Autodesk Inventor part; units mm, degrees
ref_plane "YZ Plane" through (0, 0, 0) normal (1, 0, 0) x (0, 1, 0)
ref_plane "XZ Plane" through (0, 0, 0) normal (0, 1, 0) x (-1, 0, 0)
ref_plane "XY Plane" through (0, 0, 0) normal (0, 0, 1) x (1, 0, 0)
sketch "Sketch1" plane through (0, 0, 0) normal (0, 0, 1) x (1, 0, 0)
  circle A0 centre (0, 0) radius 7.5
  line L0 (-16, 7.5) -> (16, 7.5)
  line L1 (16, 7.5) -> (16, -9.5)
  line L2 (16, -9.5) -> (-16, -9.5)
  line L3 (-16, -9.5) -> (-16, 7.5)
  line L4 (-7.5, 0) -> (-7.5, 7.5)
  line L5 (7.5, 0) -> (7.5, 7.5)
  point P0 (0, -9.5)
  dimension "d0" = 15
  dimension "d5" = 32
  dimension "d6" = 2
extrude "Extrusion1" add sketch "Sketch1" along normal blind 24.2 contours A0 L5 L0 L1 L2 L3 L4
sketch "Sketch2" plane through (0, 0, 24.2) normal (0, 0, 1) x (1, 0, 0)
  line L0 (-16, -9.5) -> (16, -9.5)
  line L1 (16, -9.5) -> (16, 7.5)
  line L2 (16, 7.5) -> (7.5, 7.5)
  line L3 (7.5, 7.5) -> (7.5, 0)
  arc A0 (-7.5, 0) -> (7.5, 0) centre (0, 0) ccw
  line L4 (-7.5, 0) -> (-7.5, 7.5)
  line L5 (-7.5, 7.5) -> (-16, 7.5)
  line L6 (-16, 7.5) -> (-16, -9.5)
  circle A1 centre (0, 0) radius 4.25
  line L7 (-7.5, 7.5) -> (-16, 7.5)
  line L8 (-7.5, 7.5) -> (7.5, 7.5)
  dimension "d10" = 8.5
extrude "Extrusion3" add sketch "Sketch2" along normal blind 3
sketch "Sketch4" plane through (0, 0, 0) normal (0, 0, -1) x (-1, 0, 0)
  line L0 (-16, 7.5) -> (-7.5, 7.5)
  line L1 (-16, -9.5) -> (-16, 7.5)
  line L2 (16, -9.5) -> (-16, -9.5)
  line L3 (16, 7.5) -> (16, -9.5)
  line L4 (7.5, 7.5) -> (16, 7.5)
  line L5 (-7.5, 7.5) -> (7.5, 7.5)
  circle A0 centre (0, 0) radius 4.25
extrude "Extrusion4" add sketch "Sketch4" along normal blind 3
sketch "Sketch5" plane through (0, 0, -3) normal (0, 0, -1) x (-1, 0, 0)
  line L0 (16, 7.5) -> (-16, 7.5)
  line L1 (16, -9.5) -> (16, 7.5)
  line L2 (-16, -9.5) -> (16, -9.5)
  line L3 (-16, 7.5) -> (-16, -9.5)
  circle A0 centre (0, 0) radius 7.5
  arc A1 (-7.5, 0) -> (7.5, 0) centre (0, 0) ccw
  line L4 (7.5, 0) -> (7.5, 7.5)
  line L5 (-16, 7.5) -> (16, 7.5)
  line L6 (-7.5, 7.5) -> (-7.5, 0)
  line L7 (-7.5, 0) -> (-7.5, 7.5)
extrude "Extrusion5" add sketch "Sketch5" along normal blind 130 contours L1 L2 L3 L0 L6 A0 L4
sketch "Sketch6" plane through (0, 0, -133) normal (0, 0, -1) x (-1, 0, 0)
  line L0 (0, 0) -> (0, -9.5) construction
  line L1 (16, -9.5) -> (-16, -9.5) construction
  line L2 (-16, 7.5) -> (-16, -9.5) construction
  point P0 (-12.5, -6)
  point P1 (12.5, -6)
  dimension "d17" = 3.5
  dimension "d18" = 3.5
hole "Hole1" at (12.5, -6, -133) at (-12.5, -6, -133) direction (0, 0, 1) diameter 2.3813 depth 10 tip angle 118
sketch "Sketch7" plane through (-16, 7.5, 27.2) normal (0, 1, 0) x (1, 0, 0)
  line L0 (16, 0) -> (16, 160.2) construction
  line L1 (32, 160.2) -> (0, 160.2)
  line L2 (0, 160.2) -> (0, 0)
  line L3 (32, 0) -> (0, 0)
  point P0 (16, 27.2)
  point P1 (3.5, 3.5)
  point P2 (3.5, 33.5)
  point P3 (3.5, 63.5)
  point P4 (3.5, 93.5)
  point P5 (3.5, 123.5)
  point P6 (3.5, 145.2)
  point P7 (28.5, 3.5)
  point P8 (28.5, 33.5)
  point P9 (28.5, 63.5)
  point P10 (28.5, 93.5)
  point P11 (28.5, 123.5)
  point P12 (28.5, 145.2)
  dimension "d27" = 3.5
  dimension "d44" = 30
  dimension "d49" = 3.5
  dimension "d50" = 15
hole "Hole3" at (-12.5, 7.5, 23.7) at (-12.5, 7.5, -6.3) at (-12.5, 7.5, -36.3) at (-12.5, 7.5, -66.3) at (-12.5, 7.5, -96.3) at (-12.5, 7.5, -118) at (12.5, 7.5, 23.7) at (12.5, 7.5, -6.3) at (12.5, 7.5, -36.3) at (12.5, 7.5, -66.3) at (12.5, 7.5, -96.3) at (12.5, 7.5, -118) direction (0, -1, 0) diameter 3.175 end through all
sketch "Sketch8" plane through (-16, -9.5, 27.2) normal (0, -1, 0) x (1, 0, 0)
  circle A0 centre (28.5, -3.5) radius 1.5875
  line L0 (30.2321, -6.5) -> (26.7679, -6.5)
  line L1 (26.7679, -6.5) -> (25.0359, -3.5)
  line L2 (25.0359, -3.5) -> (26.7679, -0.5)
  line L3 (26.7679, -0.5) -> (30.2321, -0.5)
  line L4 (30.2321, -0.5) -> (31.9641, -3.5)
  line L5 (31.9641, -3.5) -> (30.2321, -6.5)
  line L6 (5.2321, -6.5) -> (1.7679, -6.5)
  line L7 (1.7679, -0.5) -> (5.2321, -0.5)
  line L8 (5.2321, -0.5) -> (6.9641, -3.5)
  line L9 (6.9641, -3.5) -> (5.2321, -6.5)
  line L10 (1.7679, -6.5) -> (0.0359, -3.5)
  line L11 (0.0359, -3.5) -> (1.7679, -0.5)
  line L12 (0, 0) -> (0, -160.2)
  line L13 (1.7679, -36.5) -> (0.0359, -33.5)
  line L14 (0.0359, -33.5) -> (1.7679, -30.5)
  line L15 (1.7679, -30.5) -> (5.2321, -30.5)
  line L16 (5.2321, -30.5) -> (6.9641, -33.5)
  line L17 (6.9641, -33.5) -> (5.2321, -36.5)
  line L18 (25.0359, -33.5) -> (26.7679, -30.5)
  line L19 (26.7679, -36.5) -> (25.0359, -33.5)
  line L20 (30.2321, -36.5) -> (26.7679, -36.5)
  line L21 (31.9641, -33.5) -> (30.2321, -36.5)
  line L22 (30.2321, -30.5) -> (31.9641, -33.5)
  line L23 (26.7679, -30.5) -> (30.2321, -30.5)
  line L24 (1.7679, -66.5) -> (0.0359, -63.5)
  line L25 (0.0359, -63.5) -> (1.7679, -60.5)
  line L26 (1.7679, -60.5) -> (5.2321, -60.5)
  line L27 (5.2321, -60.5) -> (6.9641, -63.5)
  line L28 (6.9641, -63.5) -> (5.2321, -66.5)
  line L29 (25.0359, -63.5) -> (26.7679, -60.5)
  line L30 (26.7679, -66.5) -> (25.0359, -63.5)
  line L31 (30.2321, -66.5) -> (26.7679, -66.5)
  line L32 (31.9641, -63.5) -> (30.2321, -66.5)
  line L33 (30.2321, -60.5) -> (31.9641, -63.5)
  line L34 (26.7679, -60.5) -> (30.2321, -60.5)
  line L35 (1.7679, -96.5) -> (0.0359, -93.5)
  line L36 (0.0359, -93.5) -> (1.7679, -90.5)
  line L37 (1.7679, -90.5) -> (5.2321, -90.5)
  line L38 (5.2321, -90.5) -> (6.9641, -93.5)
  line L39 (6.9641, -93.5) -> (5.2321, -96.5)
  line L40 (25.0359, -93.5) -> (26.7679, -90.5)
  line L41 (26.7679, -96.5) -> (25.0359, -93.5)
  line L42 (30.2321, -96.5) -> (26.7679, -96.5)
  line L43 (31.9641, -93.5) -> (30.2321, -96.5)
  line L44 (30.2321, -90.5) -> (31.9641, -93.5)
  line L45 (26.7679, -90.5) -> (30.2321, -90.5)
  line L46 (1.7679, -126.5) -> (0.0359, -123.5)
  line L47 (0.0359, -123.5) -> (1.7679, -120.5)
  line L48 (1.7679, -120.5) -> (5.2321, -120.5)
  line L49 (5.2321, -120.5) -> (6.9641, -123.5)
  line L50 (6.9641, -123.5) -> (5.2321, -126.5)
  line L51 (25.0359, -123.5) -> (26.7679, -120.5)
  line L52 (26.7679, -126.5) -> (25.0359, -123.5)
  line L53 (30.2321, -126.5) -> (26.7679, -126.5)
  line L54 (31.9641, -123.5) -> (30.2321, -126.5)
  line L55 (30.2321, -120.5) -> (31.9641, -123.5)
  line L56 (26.7679, -120.5) -> (30.2321, -120.5)
  line L57 (5.2321, -36.5) -> (1.7679, -36.5)
  line L58 (5.2321, -66.5) -> (1.7679, -66.5)
  line L59 (5.2321, -96.5) -> (1.7679, -96.5)
  line L60 (5.2321, -126.5) -> (1.7679, -126.5)
  line L61 (30.2321, -148) -> (26.7679, -148)
  line L62 (31.9641, -145) -> (30.2321, -148)
  line L63 (30.2321, -142) -> (31.9641, -145)
  line L64 (26.7679, -142) -> (30.2321, -142)
  line L65 (25.0359, -145) -> (26.7679, -142)
  line L66 (26.7679, -148) -> (25.0359, -145)
  line L67 (5.2321, -142) -> (6.9641, -145)
  line L68 (6.9641, -145) -> (5.2321, -148)
  line L69 (5.2321, -148) -> (1.7679, -148)
  line L70 (1.7679, -148) -> (0.0359, -145)
  line L71 (0.0359, -145) -> (1.7679, -142)
  line L72 (1.7679, -142) -> (5.2321, -142)
  point P0 (16, -27.2)
  point P1 (1.7679, -126.5)
  point P2 (5.2321, -126.5)
  dimension "d58" = 6
  dimension "d61" = 25
  dimension "d68" = 30
  dimension "d75" = 30
  dimension "d82" = 21.5
extrude "Extrusion6" cut sketch "Sketch8" against normal blind 4 contours A0 | L0 L1 L2 L3 L4 L5 | L6 L10 L11 L7 L8 L9 | L13 L14 L15 L16 L17 L57 | L18 L23 L22 L21 L20 L19 | L24 L25 L26 L27 L28 L58 | L29 L34 L33 L32 L31 L30 | L35 L36 L37 L38 L39 L59 | L40 L45 L44 L43 L42 L41 | L46 L47 L48 L49 L50 L60 | L51 L56 L55 L54 L53 L52 | L61 L66 L65 L64 L63 L62 | L67 L68 L69 L70 L71 L72
sketch "Sketch9" plane through (0, 0, -133) normal (0, 0, -1) x (-1, 0, 0)
  line L0 (-15.9641, -9.5) -> (-15.9641, -5.5)
  line L1 (16, 7.5) -> (16, -9.5)
  line L2 (-15.9641, -9.5) -> (16, -9.5)
  line L3 (16, -9.5) -> (16, 7.5)
  line L4 (16, 7.5) -> (-15.9641, 7.5)
  line L5 (-15.9641, 7.5) -> (-15.9641, -9.5)
  point P0 (0, 0)
extrude "Extrusion7" add sketch "Sketch9" along normal blind 50
fillet "Fillet1" radius 10 2 edges at (15.9641, -1, -183) (-16, -1, -183)
sketch "Sketch10" plane through (-16, 7.5, 27.2) normal (0, 1, 0) x (1, 0, 0)
  line L0 (10, 210.2) -> (21.9641, 210.2)
  point P0 (16, 27.2)
  point P1 (15.9821, 195.2)
  point P2 (15.9821, 210.2)
  point P3 (15.9821, 210.2)
  dimension "d94" = 15
hole "Hole4" at (-0.0179, 7.5, -168) direction (0, -1, 0) diameter 15 end through all
sketch "Sketch11" plane through (-16, 7.5, 27.2) normal (0, 1, 0) x (1, 0, 0)
  line L0 (28.5, 160.2) -> (3.5, 160.2)
  line L1 (3.5, 160.2) -> (3.5, 163.2)
  line L2 (3.5, 163.2) -> (28.5, 163.2)
  line L3 (28.5, 163.2) -> (28.5, 160.2)
  line L4 (8.5, 160.2) -> (23.5, 160.2)
  point P0 (16, 27.2)
  point P1 (3.5, 161.7)
  point P2 (16, 160.2)
  dimension "d102" = 25
  dimension "d103" = 3
extrude "Extrusion8" cut sketch "Sketch11" against normal blind 15
sketch "Sketch12" plane through (-12.5, 7.5, -136) normal (0, 0, 1) x (1, 0, 0)
  line L0 (-20.042, -34.0875) -> (45.042, -34.0875)
  line L1 (45.042, -34.0875) -> (45.042, 19.0875)
  line L2 (45.042, 19.0875) -> (-20.042, 19.0875)
  line L3 (-20.042, 19.0875) -> (-20.042, -34.0875)
  line L4 (-20.042, -34.0875) -> (45.042, 19.0875) construction
  line L5 (45.042, -34.0875) -> (-20.042, 19.0875) construction
  point P0 (12.5, -7.5)
extrude "Extrusion9" cut sketch "Sketch12" along normal through all
sketch "Sketch13" plane through (-16, 7.5, -136) normal (0, 0, 1) x (1, 0, 0)
  circle A0 centre (16, -7.5) radius 4
  dimension "d108" = 8
extrude "Extrusion10" cut sketch "Sketch13" against normal blind 10
sketch "Sketch14" plane through (-6, 7.5, -183) normal (0, 1, 0) x (1, 0, 0)
  circle A0 centre (5.9821, -39.5797) radius 1.5875
  point P0 (6, -183)
  dimension "d111" = 3.175
extrude "Extrusion11" cut sketch "Sketch14" against normal blind 10
properties part number "sujecion_v3"
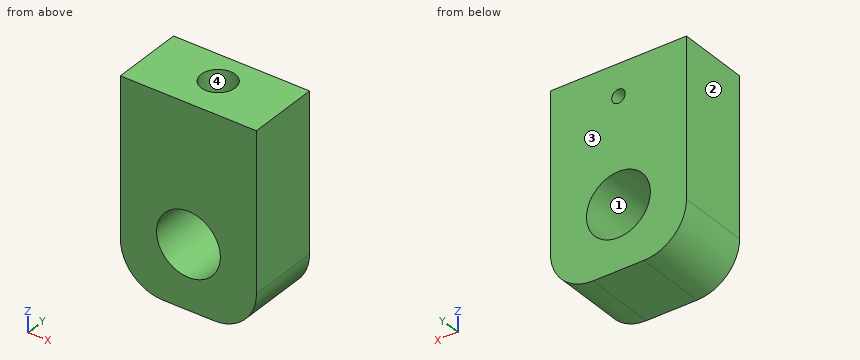
The model under review builds one solid part; all positions refer to its coordinate system, in mm. Face numbers are marked on the shaded views. Give positions to 0.01 mm unless a question says otherwise; leave off trailing zeros. Loops run counter-clockwise (first coordinate to the right, second up) from the corner with the lowest first, then second, coordinate; pieces in that order, holes last. Notation, with made-up numbers: (86.5, -1) -> (113.5, -1) arc R32 cw to (113.5, 27) -> close; hole circle Ø1 at (-2.75, -14). An arc over 180 degrees is marked (long way). Put each result on its own line as item: value. Start each with the question number.
1. Wall thickness on probe 1 along Y at (x, z) = (0, -140.25); probe 2 along Z at (x, y) = (0, -6.25); probe 3 along X at (y, z) = (3.25, -168): over which ranges is each line inside the solid? List them lowest first.
2. We need section A-A on z = -168. State the section outline as (x, y) points.
3. We need section B-B on x = 3. State the section outline as (y, z) points, then the cut area to 3 significant figures.
4. We need section D-D on z = -175. State the section outline as (x, y) points, then the cut area to 3 significant figures.
5. Mouldability with a two-part tool opening along X and no side actions: class the marked faces 1, 2, 3 and 4 as released by +X, released by -X, zero draft, split by the parting line, or undercut.
6. We need section C-C on y = -1.75. State the section outline as (x, z) points.
7. Clearance check with a flat-ended pin moving along its axis: P1, Ø4, axis at x = -0.5, y = 1.5, coming from the +Z side. State where the tip first meets the part, or that it passes through.
Determined:
1. probe 1: -9.5 to -4, 4 to 7.5
1. probe 2: -183 to -175.5, -160.5 to -136
1. probe 3: -16 to -7.52, 7.48 to 15.96
2. outline: (-16, -9.5) -> (-7.52, -9.5) -> (-7.52, 7.5) -> (-16, 7.5) -> close; (7.48, -9.5) -> (15.96, -9.5) -> (15.96, 7.5) -> (7.48, 7.5) -> close
3. outline: (-9.5, -183) -> (7.5, -183) -> (7.5, -174.87) -> (-9.5, -174.87) -> close; (-9.5, -161.13) -> (7.5, -161.13) -> (7.5, -136) -> (2.65, -136) -> (2.65, -146) -> (-2.65, -146) -> (-2.65, -136) -> (-9.5, -136) -> close
3. area: 513 mm^2
4. outline: (-15.8, -9.5) -> (-2.71, -9.5) -> (-2.71, 7.5) -> (-15.8, 7.5) -> close; (2.67, -9.5) -> (15.76, -9.5) -> (15.76, 7.5) -> (2.67, 7.5) -> close
4. area: 445 mm^2
5. face 1: undercut
5. face 2: released by -X
5. face 3: zero draft
5. face 4: undercut
6. outline: (-16, -173) arc R10 ccw to (-6, -183) -> (5.96, -183) arc R10 ccw to (15.96, -173) -> (15.96, -136) -> (3.6, -136) -> (3.6, -146) -> (-3.6, -146) -> (-3.6, -136) -> (-16, -136) -> close; hole circle Ø15 at (-0.02, -168)
7. P1: z = -146
